The listing builds one solid part. Answer for the finished solid, in the listing's coordinates (mm). A direction names the side the tool comes from. Give positions to 0.01 mm unless a question says otherwise; leave off trailing zeros. Order: outer loops, then holes, each group sorted by start corner. A loop starts at its lowest first (then second) coordinate and runs counter-clockwise, first axis right, second up. Notation, with made-up numbers: (-6.75, -6.75) - (39.25, -6.75) arc R21 ccw to (39.25, 9.25) - close; hole circle Ø7 at (87, -36). An arc over 180 degrees is marked (long way). Answer in a Markdown table with one row per item.
from build123d import *

# Parameters (mm, degrees)
SKETCH1_W           = 10
SKETCH1_H           = 2.5
SKETCH1_W_2         = 38
SKETCH1_H_2         = 5
BOSS_EXTRUDE1_DEPTH = 1.25


with BuildPart() as part:
    # Sketch1 → Boss-Extrude1 (new, symmetric)
    with BuildSketch(Plane(origin=(0, 0, 0), x_dir=(0, 0, -1), z_dir=(1, 0, 0))):
        Polygon((-77.50700933, 25), (-77.50700933, -25), (-57.50700933, -25), (-57.50700933, -30), (-42.50700933, -30), (-42.50700933, -25), (-22.50700933, -25), (-22.50700933, -30), (-7.50700933, -30), (-7.50700933, -25), (7.50700933, -25), (7.50700933, -30), (22.50700933, -30), (22.50700933, -25), (42.50700933, -25), (42.50700933, -30), (57.50700933, -30), (57.50700933, -25), (77.50700933, -25), (77.50700933, 25), (57.50700933, 25), (57.50700933, 27.5), (42.50700933, 27.5), (42.50700933, 25), (22.50700933, 25), (22.50700933, 27.5), (7.50700933, 27.5), (7.50700933, 25), (-7.50700933, 25), (-7.50700933, 27.5), (-22.50700933, 27.5), (-22.50700933, 25), (-42.50700933, 25), (-42.50700933, 27.5), (-57.50700933, 27.5), (-57.50700933, 25), align=None)
        with Locations((0, 17.5)):
            Rectangle(SKETCH1_W, SKETCH1_H, mode=Mode.SUBTRACT)
        with Locations((-46, -8.75)):
            Rectangle(SKETCH1_W_2, SKETCH1_H_2, mode=Mode.SUBTRACT)
        with Locations((0, -17.5)):
            Rectangle(SKETCH1_W, SKETCH1_H, mode=Mode.SUBTRACT)
        with Locations((-20, -17.5)):
            Rectangle(SKETCH1_W, SKETCH1_H, mode=Mode.SUBTRACT)
        with Locations((-20, 17.5)):
            Rectangle(SKETCH1_W, SKETCH1_H, mode=Mode.SUBTRACT)
        with Locations((-40, -17.5)):
            Rectangle(SKETCH1_W, SKETCH1_H, mode=Mode.SUBTRACT)
        with Locations((-40, 17.5)):
            Rectangle(SKETCH1_W, SKETCH1_H, mode=Mode.SUBTRACT)
        with Locations((-60, -17.5)):
            Rectangle(SKETCH1_W, SKETCH1_H, mode=Mode.SUBTRACT)
        with Locations((-60, 17.5)):
            Rectangle(SKETCH1_W, SKETCH1_H, mode=Mode.SUBTRACT)
        with Locations((20, -17.5)):
            Rectangle(SKETCH1_W, SKETCH1_H, mode=Mode.SUBTRACT)
        with Locations((20, 17.5)):
            Rectangle(SKETCH1_W, SKETCH1_H, mode=Mode.SUBTRACT)
        with Locations((40, -17.5)):
            Rectangle(SKETCH1_W, SKETCH1_H, mode=Mode.SUBTRACT)
        with Locations((40, 17.5)):
            Rectangle(SKETCH1_W, SKETCH1_H, mode=Mode.SUBTRACT)
        with Locations((60, -17.5)):
            Rectangle(SKETCH1_W, SKETCH1_H, mode=Mode.SUBTRACT)
        with Locations((60, 17.5)):
            Rectangle(SKETCH1_W, SKETCH1_H, mode=Mode.SUBTRACT)
        with Locations((0, 8.75)):
            Rectangle(SKETCH1_W_2, SKETCH1_H_2, mode=Mode.SUBTRACT)
        with Locations((46, 8.75)):
            Rectangle(SKETCH1_W_2, SKETCH1_H_2, mode=Mode.SUBTRACT)
        with Locations((-46, 0)):
            Rectangle(SKETCH1_W_2, SKETCH1_H_2, mode=Mode.SUBTRACT)
        with Locations((-46, 8.75)):
            Rectangle(SKETCH1_W_2, SKETCH1_H_2, mode=Mode.SUBTRACT)
        with Locations((46, -8.75)):
            Rectangle(SKETCH1_W_2, SKETCH1_H_2, mode=Mode.SUBTRACT)
        with Locations((46, 0)):
            Rectangle(SKETCH1_W_2, SKETCH1_H_2, mode=Mode.SUBTRACT)
        Rectangle(SKETCH1_W_2, SKETCH1_H_2, mode=Mode.SUBTRACT)
        with Locations((0, -8.75)):
            Rectangle(SKETCH1_W_2, SKETCH1_H_2, mode=Mode.SUBTRACT)
    extrude(amount=BOSS_EXTRUDE1_DEPTH, both=True)


solid = part.part
Item 1: Each of these flat-tipped pins is pushed along its axis until it touches: P1, Ø0.8, axis at x = 0, z = -62, coming from the +Y side; P2, Ø0.8, axis at x = -0.5, y = 25.5, coming from the -Z side. Where does it stop, or does it pass through?
Answer block:
| item | result |
|---|---|
| P1 | y = 25 |
| P2 | z = -57.51 |
Item 2: Find section A-A on z = -52. Write down the section's boundary in (x, y), then the cut area to 3 significant figures.
Answer block:
| item | result |
|---|---|
| outline | (-1.25, -30) - (1.25, -30) - (1.25, -11.25) - (-1.25, -11.25) - close; (-1.25, -6.25) - (1.25, -6.25) - (1.25, -2.5) - (-1.25, -2.5) - close; (-1.25, 2.5) - (1.25, 2.5) - (1.25, 6.25) - (-1.25, 6.25) - close; (-1.25, 11.25) - (1.25, 11.25) - (1.25, 27.5) - (-1.25, 27.5) - close |
| area | 106 mm² |
Item 3: Find section B-B on y = 8. Write down the section's boundary in (x, z).
Answer block:
| item | result |
|---|---|
| outline | (-1.25, -77.51) - (1.25, -77.51) - (1.25, -65) - (-1.25, -65) - close; (-1.25, -27) - (1.25, -27) - (1.25, -19) - (-1.25, -19) - close; (-1.25, 19) - (1.25, 19) - (1.25, 27) - (-1.25, 27) - close; (-1.25, 65) - (1.25, 65) - (1.25, 77.51) - (-1.25, 77.51) - close |
Item 4: Consider line 1 (Z direction, x = -0.75, y = -26); line 2 (Y direction, x = -0.4, z = 17.5); line 3 (Y direction, x = -0.05, z = -0.5). Determine where each line is inside the solid, lowest interval first.
Answer block:
| item | result |
|---|---|
| line 1 | -57.51 to -42.51, -22.51 to -7.51, 7.51 to 22.51, 42.51 to 57.51 |
| line 2 | -30 to -18.75, -16.25 to -11.25, -6.25 to -2.5, 2.5 to 6.25, 11.25 to 16.25, 18.75 to 27.5 |
| line 3 | -25 to -18.75, -16.25 to -11.25, -6.25 to -2.5, 2.5 to 6.25, 11.25 to 16.25, 18.75 to 25 |
Item 5: Find section C-C on z = -16.5. Write down the section's boundary in (x, y), then the cut area to 4 significant figures.
Answer block:
| item | result |
|---|---|
| outline | (-1.25, -30) - (1.25, -30) - (1.25, -18.75) - (-1.25, -18.75) - close; (-1.25, -16.25) - (1.25, -16.25) - (1.25, -11.25) - (-1.25, -11.25) - close; (-1.25, -6.25) - (1.25, -6.25) - (1.25, -2.5) - (-1.25, -2.5) - close; (-1.25, 2.5) - (1.25, 2.5) - (1.25, 6.25) - (-1.25, 6.25) - close; (-1.25, 11.25) - (1.25, 11.25) - (1.25, 16.25) - (-1.25, 16.25) - close; (-1.25, 18.75) - (1.25, 18.75) - (1.25, 27.5) - (-1.25, 27.5) - close |
| area | 93.75 mm² |
Item 6: Determine the mould class of faces 1 (the face through (0, -25, -67)), 2 (the face through (0, -18, 15)) for opening direction Z: pulls with the +Z half, pulls with the -Z half, needs draft (parallel to the pull), parting line crosses it, or undercut.
Answer block:
| item | result |
|---|---|
| face 1 | needs draft |
| face 2 | undercut |
Item 7: Which of the six approach directions +Z, -Z, +X, -X, +Y, -Y give full straight-line access (tool end or side, diameter ignored) to faces 3 (the face through (0, 26, 22.507)), 4 (the face through (0, -25, 33)), 5 (the face through (0, -6.25, 0))?
Answer block:
| item | result |
|---|---|
| face 3 | +X, -X, +Y |
| face 4 | +X, -X, -Y |
| face 5 | +X, -X |
Item 8: Find section D-D on x = -0.6. Count the separate pieces of the cut face and the enclosed holes in it, then the cut area to 3 significant figures.
Answer block:
| item | result |
|---|---|
| separate pieces | 1 |
| enclosed holes | 23 |
| area | 6,140 mm² |
